Geometry: final body of the model. Coordinates: model frame, mm. A direction names the side the tool comes from. Give positions to 0.01 mm unless a question says otherwise; leave off trailing zeros. Order: outer loops, then holes, each group sorted by start corner. A loop starts at its lowest first (then second) coordinate and runs counter-clockwise, first axis right, second up. Notation, with made-up numbers: (2.5, 75.5) -> (14.5, 75.5) arc R21 cw to (14.5, 103.5) -> close; hole circle Ø8 at (29, -21.75). An arc over 180 degrees is marked (long way). Answer in a Markdown table with one row per item. Add a question column.
Q1. Line query: line 1 along X through (y, z) = (-16.5, 25); line 2 along Y through (x, z) = (82.5, 25.5); line 3 along Z through (x, y) = (49.5, 1). Output: solid intervals per line, ascending. Write a range as from..to.
Q2. Pull-direction query (Y, two-part tool) for faces 1 (the face through (119.25, -21.23, 30.62)), 2 (the face through (119.25, -5.23, 30.62)), 3 (the face through (52.53, 1.97, 20.56)), 4 (the face through (81, 4, 29)); classes: +Y half, -Y half, draft (parallel to the pull), parting line (faces both ways), or undercut.
Q3. Cut plane D-D on y = 2.5. Return the cut outline in (x, z), and give its area (3 significant figures).
Q4. Cut plane B-B on z = 39.5. Return the cut outline in (x, y).
Q5. Cut plane C-C on y = -22. Return the cut outline in (x, z).
Q6. Cut plane A-A on z = 24.5. Return the cut outline in (x, y).
Q7. Set-up query: faces 5 (the face through (25.555, 1.972, 41.719)), 6 (the face through (118, -6, 22.493)), 7 (the face through (75.3, 0, 30.7)). Return all of +Z, -Z, +X, -X, +Y, -Y with unobstructed straight access to the full face (end or side cutting, diameter ignored); none if empty.
Q8. Contact query for flat-ended pins moving along their axis: P1, Ø6, axis at y = -25, z = 40, coming from the -X side; P2, Ø1, axis at x = 101.5, z = 27.5, coming from the -Y side; P3, Ø4, axis at x = 23.78, z = 40.59, coming from the -Y side; P4, Ø6.5, axis at x = 67.28, z = 25.34, coming from the +Y side. Output: stop coordinate, or through.
from build123d import *

# Parameters (mm, degrees)
SKETCH1_R           = 2.1
BOSS_EXTRUDE1_DEPTH = 4
SKETCH3_W           = 30
SKETCH3_H           = 34
BOSS_EXTRUDE4_DEPTH = 4
SKETCH4_R           = 2.1
CUT_EXTRUDE1_DEPTH  = 4


with BuildPart() as part:
    # Sketch1 → Boss-Extrude1 (new body)
    with BuildSketch(Plane(origin=(0, 0, 0), x_dir=(1, 0, 0), z_dir=(0, 1, 0))):
        with BuildLine():
            Line((19.185222031, -38.125659411), (19.185222031, -50.522227261))
            ThreePointArc((19.185222031, -50.522227261), (68.648777269, -30.725135996), (117.277214352, -52.493076326))
            Line((117.277214352, -52.493076326), (117.277214352, -22.493076326))
            Line((117.277214352, -22.493076326), (89.144688482, -22.493076326))
            ThreePointArc((89.144688482, -22.493076326), (52.012033316, -20.674538522), (19.185222031, -38.125659411))
        make_face()
        with Locations(Location((67.277214352, -25.33669757, 0), (0, 0, 270))):
            Circle(SKETCH1_R, mode=Mode.SUBTRACT)
        with Locations(Location((23.784262782, -40.590182935, 0), (0, 0, 270))):
            Circle(SKETCH1_R, mode=Mode.SUBTRACT)
        with Locations(Location((110.770165922, -40.590182935, 0), (0, 0, 90))):
            Circle(SKETCH1_R, mode=Mode.SUBTRACT)
    extrude(amount=BOSS_EXTRUDE1_DEPTH)

    # Sketch3 → Boss-Extrude4 (add)
    with BuildSketch(Plane(origin=(117.277214352, 0, 0), x_dir=(0, 0, -1), z_dir=(1, 0, 0))):
        with Locations((-37.493076326, -13)):
            Rectangle(SKETCH3_W, SKETCH3_H)
    extrude(amount=BOSS_EXTRUDE4_DEPTH)

    # Sketch4 → Cut-Extrude1 (cut)
    with BuildSketch(Plane.ZY.offset(-117.277214352)):
        with Locations((29.492163097, -6.999086771)):
            Circle(SKETCH4_R)
        with Locations((45.493989555, -6.999086771)):
            Circle(SKETCH4_R)
        with Locations((45.493989555, -23.000913229)):
            Circle(SKETCH4_R)
        with Locations((29.492163097, -23.000913229)):
            Circle(SKETCH4_R)
    extrude(amount=-CUT_EXTRUDE1_DEPTH, mode=Mode.SUBTRACT)


solid = part.part
Completed:
| question | item | result |
|---|---|---|
| 1 | line 1 | x = 117.28..121.28 |
| 1 | line 2 | y = 0..4 |
| 1 | line 3 | z = 21.28..33.07 |
| 2 | face 1 | undercut |
| 2 | face 2 | undercut |
| 2 | face 3 | draft |
| 2 | face 4 | +Y half |
| 3 | outline | (19.19, 38.13) arc R70 ccw to (89.14, 22.49) -> (121.28, 22.49) -> (121.28, 52.49) -> (117.28, 52.49) arc R68.28 cw to (19.19, 50.52) -> close; hole circle Ø4.2 at (23.78, 40.59); hole circle Ø4.2 at (67.28, 25.34); hole circle Ø4.2 at (110.77, 40.59) |
| 3 | area | 1,450 mm² |
| 4 | outline | (19.19, 0) -> (21.99, 0) -> (21.99, 4) -> (19.19, 4) -> close; (25.58, 0) -> (33.77, 0) -> (33.77, 4) -> (25.58, 4) -> close; (100.79, 0) -> (108.98, 0) -> (108.98, 4) -> (100.79, 4) -> close; (112.57, 0) -> (117.28, 0) -> (117.28, -30) -> (121.28, -30) -> (121.28, 4) -> (112.57, 4) -> close |
| 5 | outline | (117.28, 22.49) -> (121.28, 22.49) -> (121.28, 27.65) -> (117.28, 27.65) -> close; (117.28, 31.34) -> (121.28, 31.34) -> (121.28, 43.65) -> (117.28, 43.65) -> close; (117.28, 47.34) -> (121.28, 47.34) -> (121.28, 52.49) -> (117.28, 52.49) -> close |
| 6 | outline | (40.05, 0) -> (65.35, 0) -> (65.35, 4) -> (40.05, 4) -> close; (69.2, 0) -> (117.28, 0) -> (117.28, -30) -> (121.28, -30) -> (121.28, 4) -> (69.2, 4) -> close |
| 7 | face 5 | +Y, -Y |
| 7 | face 6 | -Z, +X, +Y, -Y |
| 7 | face 7 | +Z, -Z, -X, -Y |
| 8 | P1 | stops at x = 117.28 |
| 8 | P2 | stops at y = 0 |
| 8 | P3 | passes through |
| 8 | P4 | stops at y = 4 |
